Read the model definition and answer for the solid it produces. Units are mm, in the model's axes. Round coordinates to 2 decimals unless told otherwise and drop trailing zeros. Write each loop counter-clockwise with the first axis right and the second up, starting at its lowest first coordinate (ties: lowest second). Pieces come first, ordered by that corner, then holes.
from build123d import *

# Parameters (mm, degrees)
SKICA1_W                = 72.4
SKICA1_H                = 22.9
P_IDAT_VYSUNUT_M2_DEPTH = 1.2
SKICA2_W                = 70
SKICA2_H                = 20.5
P_IDAT_VYSUNUT_M3_DEPTH = 1


with BuildPart() as part:
    # Skica1 → Přidat vysunutím2 (new body)
    with BuildSketch(Plane(origin=(0, 0, 0), x_dir=(1, 0, 0), z_dir=(0, 1, 0))):
        with Locations((36.2, 11.45)):
            Rectangle(SKICA1_W, SKICA1_H)
    extrude(amount=P_IDAT_VYSUNUT_M2_DEPTH)

    # Skica2 → Přidat vysunutím3 (add)
    with BuildSketch(Plane(origin=(0, 1.2, 0), x_dir=(1, 0, 0), z_dir=(0, 1, 0))):
        with Locations((36.2, 11.45)):
            Rectangle(SKICA2_W, SKICA2_H)
    extrude(amount=P_IDAT_VYSUNUT_M3_DEPTH)


solid = part.part
Q1. Straight lines are drawn through the part: probe 1 along Z at (x, y) = (56, 1.3); probe 2 along X at (y, z) = (1.95, -10.5); probe 3 along Y at (x, z) = (4, -22). For each, find the intervals that lie inside material, in ascending order.
Verdict:
probe 1: z = -21.7 to -1.2
probe 2: x = 1.2 to 71.2
probe 3: y = 0 to 1.2
Q2. Section B-B (z = -9.5) is taken. Determine the outline of the cut face in (x, y), then the cut area to 3 significant figures.
Verdict:
outline: (0, 0) - (72.4, 0) - (72.4, 1.2) - (71.2, 1.2) - (71.2, 2.2) - (1.2, 2.2) - (1.2, 1.2) - (0, 1.2) - close
area: 157 mm2
Q3. A flat-ended cylindrical pin translates along its axis: pin 1 Ø1.1 at (x, y) = (35, 2) entering from -Z. Find the tip coordinate at first contact, or state that the pin passes through.
Verdict:
pin 1: stops at z = -21.7
Q4. Section C-C (y = 1.6) is taken. Determine the outline of the cut face in (x, z).
Verdict:
outline: (1.2, -21.7) - (71.2, -21.7) - (71.2, -1.2) - (1.2, -1.2) - close
Q5. Section A-A (x = 40) is taken. Determine the outline of the cut face in (y, z), then the cut area to 3 significant figures.
Verdict:
outline: (0, -22.9) - (1.2, -22.9) - (1.2, -21.7) - (2.2, -21.7) - (2.2, -1.2) - (1.2, -1.2) - (1.2, 0) - (0, 0) - close
area: 48.0 mm2
